```python
from build123d import *


with BuildPart() as part:
    # 草图1 → 旋转1 (revolve)
    with BuildSketch(Plane(origin=(0, 0, 0), x_dir=(0, 0, -1), z_dir=(1, 0, 0)), mode=Mode.PRIVATE) as revolve_1_sk:
        with BuildLine():
            Line((0, 4.5), (-0.5, 4.5))
            ThreePointArc((-0.5, 4.5), (-1.560660172, 4.060660172), (-2, 3))
            Line((-2, 3), (-2, 0))
            Line((-2, 0), (7, 0))
            Line((7, 0), (7, 1.5))
            Line((7, 1.5), (4.556999532, 2.5))
            Line((4.556999532, 2.5), (4.352333177, 2))
            Line((4.352333177, 2), (3.130832943, 2.5))
            Line((3.130832943, 2.5), (2.926166589, 2))
            Line((2.926166589, 2), (1.704666355, 2.5))
            Line((1.704666355, 2.5), (1.5, 2))
            Line((1.5, 2), (0, 2))
            Line((0, 2), (0, 4.5))
        make_face()
    revolve(revolve_1_sk.sketch.rotate(Axis((0, 0, 35.672992327), (0, 0, -1)), 90), axis=Axis((0, 0, 35.672992327), (0, 0, -1)))


solid = part.part
```
The listing builds one solid part. Answer for the finished solid, in the listing's coordinates (mm). Give positions to 0.01 mm unless a question says otherwise; leave off trailing zeros. Order: outer loops, then holes, each group sorted by start corner. A loop starts at its lowest first (then second) coordinate and runs counter-clockwise, first axis right, second up. Notation, with made-up numbers: M 52.5,83.5 L 65.5,83.5 A3 ccw 65.5,87.5 Z; hole C 38.25,18 d8. An arc over 180 degrees is marked long. Put each result on its own line as item: value. Start each with the question number.
Item 1: Find the intervals of material crossed by line 1 along Z through (x, y) = (-1.25, 2.5); line 2 along Y through (x, z) = (-1.25, 0.25); line 3 along X through (y, z) = (1.75, 1.25), in increasing order.
Item 2: Flat-ended cylindrical pins translate along their axes: P1, Ø1, axis at x = -2, y = 3.5, coming from the +Z side; P2, Ø2.5, axis at x = -1, y = -2, coming from the -Z side. Find the tip coordinate at first contact, or state that the pin passes through.
Item 3: For a pull along Z with two mould halves and no side action, classify faces 1 (the face through (0, 2, -1)), 2 (the face through (-1, 2, 0)), 3 (the face through (1.596, -0.503, -6.576)), 4 (the face through (-3.32, -3.04, 0.25)) as +Z half, -Z half, draft (parallel to the pull), parting line (faces both ways), or undercut.
Item 4: The part is cut by section C-C, the plane z = -2. Determine the outline of the cut face in (x, y), and give its area (3 significant figures).
Item 5: The part is cut by section A-A, the plane x = 0. Determine the outline of the cut face in (y, z), and give its area (3 significant figures).
Answer key:
1. line 1: z = 0 to 2
1. line 2: y = -4.32 to 4.32
1. line 3: x = -3.93 to 3.93
2. P1: stops at z = 1.9
2. P2: stops at z = -7
3. face 1: undercut
3. face 2: undercut
3. face 3: -Z half
3. face 4: draft
4. outline: C 0,0 d4.76
4. area: 17.8 mm²
5. outline: M -4.5,0 L -2,0 L -2,-1.5 L -2.5,-1.7 L -2,-2.93 L -2.5,-3.13 L -2,-4.35 L -2.5,-4.56 L -1.5,-7 L 1.5,-7 L 2.5,-4.56 L 2,-4.35 L 2.5,-3.13 L 2,-2.93 L 2.5,-1.7 L 2,-1.5 L 2,0 L 4.5,0 L 4.5,0.5 A1.5 ccw 3,2 L -3,2 A1.5 ccw -4.5,0.5 Z
5. area: 46.6 mm²
